For this review, take the finished solid that the model builds, in its own axes (mm). Face numbers are marked on the shaded views. A direction names the side the tool comes from. Give positions to 0.01 mm unless a question says otherwise; leave off trailing zeros. Order: outer loops, then holes, each group sorted by start corner. A loop starts at its lowest first (then second) coordinate and runs counter-clockwise, first axis right, second up.
Item 1: For probe 1 along Y at (x, z) = (0, -24.1); probe 2 along Y at (x, z) = (0, -6.5); probe 3 along Y at (x, z) = (0, -5), list the stretches that pass through material, from the lowest coordinate up.
Item 2: Consider section D-D (z = -20.25). Give the boundary of the cut face in (x, y).
Item 3: For P1, Ø3, axis at x = -0.5, z = -3.5, coming from the -Y side; P2, Ø3, axis at x = 3.5, z = -20, coming from the -Y side; P3, Ø1.5, axis at y = 4.5, z = -18.5, coming from the -X side, all flat-tipped, find the tip position at first contact; note any pin that passes through.
Item 4: Consider section A-A (z = -4.05). Give the boundary of the cut face in (x, y), plus the area to 3 significant figures.
Item 5: Machinability: for the marked faces 4 and 5, which of the approach directions +Z, -Z, +X, -X, +Y, -Y give a long, thin tool a straight path to every point of the face, cutting with its end or side? Answer none if there is none.
Item 6: Consider section C-C (z = -9). Give the boundary of the cut face in (x, y), plus the area to 3 significant figures.
Item 7: The part is to be moulded in two halves that separate along X. For the marked faces 1, 2 and 3, say which applies: released by +X, released by -X, zero draft, split by the parting line, or undercut.
Item 8: Consider section B-B (z = -24.75). Give the boundary of the cut face in (x, y).
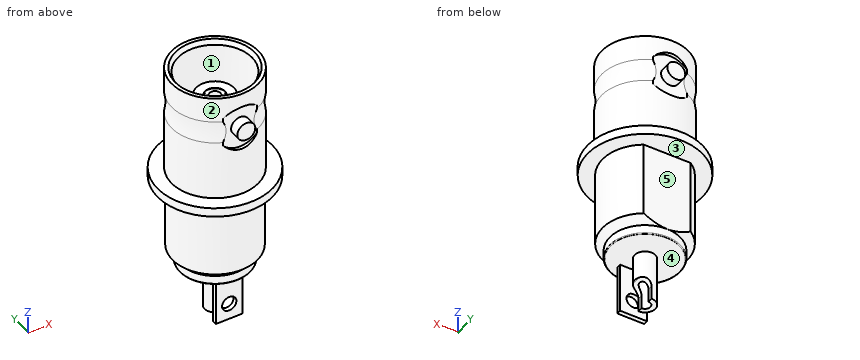
```python
from build123d import *

# Parameters (mm, degrees)
CUT_EXTRUDE_START        = 4.4
SKETCH_3_R               = 2.5
CUT_EXTRUDE_2_DEPTH      = 21.197865761
CUT_EXTRUDE_START_2      = -4.4
SKETCH_3_2_R             = 2.5
CUT_EXTRUDE_3_DEPTH      = 21.197865761
EXTRUDE_START            = 4.4
SKETCH_5_R               = 1
EXTRUDE_4_DEPTH          = 1.1
EXTRUDE_START_2          = -5.5
SKETCH_5_2_R             = 1
EXTRUDE_5_DEPTH          = 1.1
CUT_EXTRUDE_6_DEPTH      = 10
SKETCH_7_R               = 1.15
SKETCH_7_R_2             = 0.6
SKETCH_7_W               = 3
SKETCH_7_H               = 0.5
EXTRUDE_8_DEPTH          = 5.5
CUT_EXTRUDE_9_DEPTH      = 1.5
CUT_EXTRUDE_9_DEPTH_BACK = 1.5
SKETCH_9_R               = 0.8
CUT_EXTRUDE_10_DEPTH     = 1


with BuildPart() as part:
    # Эскиз1 → Повернуть1 (revolve)
    with BuildSketch(Plane(origin=(0, 0, 0), x_dir=(0, 0, -1), z_dir=(1, 0, 0)), mode=Mode.PRIVATE) as revolve_1_sk:
        with BuildLine():
            Line((10.3, 0), (10.3, 0.6))
            Line((10.3, 0.6), (3.3, 0.6))
            Line((3.3, 0.6), (3.3, 1))
            ThreePointArc((3.3, 1), (3.35, 1.05), (3.3, 1.1))
            Line((3.3, 1.1), (3.3, 2.1))
            Line((3.3, 2.1), (8.4, 2.1))
            Line((8.4, 2.1), (8.4, 4.1))
            Line((8.4, 4.1), (0.5, 4.1))
            Line((0.5, 4.1), (0, 4.4))
            Line((0, 4.4), (0, 4.8))
            Line((0, 4.8), (2.8, 4.8))
            ThreePointArc((2.8, 4.8), (4.05, 4.668347297), (5.3, 4.8))
            Line((5.3, 4.8), (11.9, 4.8))
            Line((11.9, 4.8), (11.9, 6.35))
            Line((11.9, 6.35), (12.9, 6.35))
            Line((12.9, 6.35), (12.9, 4.7))
            Line((12.9, 4.7), (21.1, 4.7))
            Line((21.1, 4.7), (21.9, 3.9))
            Line((21.9, 3.9), (22.8, 3.9))
            ThreePointArc((22.8, 3.9), (22.870710678, 3.870710678), (22.9, 3.8))
            Line((22.9, 3.8), (22.9, 0))
            Line((22.9, 0), (10.3, 0))
        make_face()
    revolve(revolve_1_sk.sketch.rotate(Axis((0, 0, 0), (0, 0, -1)), 90), axis=Axis((0, 0, 0), (0, 0, -1)))

    # Эскиз3 → Вытянуть2 (cut, through all)
    with BuildSketch(Plane(origin=(0, 0, 0), x_dir=(1, 0, 0), z_dir=(0, 1, 0)).offset(CUT_EXTRUDE_START)):
        with Locations((0, 4.05)):
            Circle(SKETCH_3_R)
    extrude(amount=CUT_EXTRUDE_2_DEPTH, mode=Mode.SUBTRACT)

    # Эскиз3<2> → Вытянуть3 (cut, through all)
    with BuildSketch(Plane(origin=(0, 0, 0), x_dir=(1, 0, 0), z_dir=(0, 1, 0)).offset(CUT_EXTRUDE_START_2)):
        with Locations((0, 4.05)):
            Circle(SKETCH_3_2_R)
    extrude(amount=-CUT_EXTRUDE_3_DEPTH, mode=Mode.SUBTRACT)

    # Эскиз5 → Вытянуть4 (add)
    with BuildSketch(Plane(origin=(0, 0, 0), x_dir=(1, 0, 0), z_dir=(0, 1, 0)).offset(EXTRUDE_START)):
        with Locations(Location((0, 4.05, 0), (0, 0, 270))):
            Circle(SKETCH_5_R)
    extrude(amount=EXTRUDE_4_DEPTH)

    # Эскиз5<2> → Вытянуть5 (add)
    with BuildSketch(Plane(origin=(0, 0, 0), x_dir=(1, 0, 0), z_dir=(0, 1, 0)).offset(EXTRUDE_START_2)):
        with Locations(Location((0, 4.05, 0), (0, 0, 270))):
            Circle(SKETCH_5_2_R)
    extrude(amount=EXTRUDE_5_DEPTH)

    # Эскиз2 → Вытянуть6 (cut)
    with BuildSketch(Plane(origin=(0, 0, -22.9), x_dir=(-1, 0, 0), z_dir=(0, 0, -1))):
        with BuildLine():
            Line((-2.62297541, 3.9), (2.62297541, 3.9))
            ThreePointArc((2.62297541, 3.9), (0, 4.7), (-2.62297541, 3.9))
        make_face()
    extrude(amount=-CUT_EXTRUDE_6_DEPTH, mode=Mode.SUBTRACT)

    # Эскиз7 → Вытянуть8 (add)
    # profile 1 of 2: a face of its own
    with BuildSketch(Plane(origin=(0, 0, -22.9), x_dir=(-1, 0, 0), z_dir=(0, 0, -1))):
        with Locations(Location((0, 0, 0), (0, 0, 180))):
            Circle(SKETCH_7_R)
        with Locations(Location((0, 0, 0), (0, 0, 180))):
            Circle(SKETCH_7_R_2, mode=Mode.SUBTRACT)
    # profile 2 of 2: a face of its own
    with BuildSketch(Plane(origin=(0, 0, -22.9), x_dir=(-1, 0, 0), z_dir=(0, 0, -1))):
        with Locations((0, -2.25)):
            Rectangle(SKETCH_7_W, SKETCH_7_H)
    extrude(amount=EXTRUDE_8_DEPTH)

    # Эскиз8 → Вытянуть9 (cut, two sides: drawn at the far end of the back side and taken through both)
    with BuildSketch(Plane(origin=(0, 0, 0), x_dir=(1, 0, 0), z_dir=(0, 1, 0)).offset(-CUT_EXTRUDE_9_DEPTH_BACK)):
        with BuildLine():
            Line((0, 30.676927372), (3.471261933, 30.676927372))
            Line((3.471261933, 30.676927372), (3.471261933, 25.9))
            Line((3.471261933, 25.9), (1, 25.9))
            ThreePointArc((1, 25.9), (0.292893219, 26.192893219), (0, 26.9))
            Line((0, 26.9), (0, 30.676927372))
        make_face()
    extrude(amount=CUT_EXTRUDE_9_DEPTH + CUT_EXTRUDE_9_DEPTH_BACK, mode=Mode.SUBTRACT)

    # Эскиз9 → Вытянуть10 (cut)
    with BuildSketch(Plane.XZ.offset(2.5)):
        with Locations((0, -26.6)):
            Circle(SKETCH_9_R)
    extrude(amount=-CUT_EXTRUDE_10_DEPTH, mode=Mode.SUBTRACT)


solid = part.part
```
Resolved:
1. probe 1: y = -2.5 to -2, -1.15 to -0.6, 0.6 to 1.15
1. probe 2: y = -4.4 to -4.1, -2.1 to -0.6, 0.6 to 2.1, 4.1 to 4.4
1. probe 3: y = -5.5 to -4.1, -2.1 to -0.6, 0.6 to 2.1, 4.1 to 5.5
2. outline: (-2.62, 3.9) arc R4.7 ccw (long way) to (2.62, 3.9) - close
3. P1: stops at y = -5.5
3. P2: stops at y = -4.25
3. P3: stops at x = -2.83
4. outline: circle Ø4.2 at (0, 0); (-1.56, -4.4) - (-1, -4.4) - (-1, -5.5) - (1, -5.5) - (1, -4.4) - (1.56, -4.4) arc R4.67 ccw to (1.56, 4.4) - (1, 4.4) - (1, 5.5) - (-1, 5.5) - (-1, 4.4) - (-1.56, 4.4) arc R4.67 ccw to start; hole circle Ø8.2 at (0, 0); hole circle Ø1.2 at (0, 0)
4. area: 31.7 mm2
5. face 4: -Z
5. face 5: -Z, +X, -X, +Y
6. outline: circle Ø9.6 at (0, 0); hole circle Ø1.2 at (0, 0)
6. area: 71.3 mm2
7. face 1: undercut
7. face 2: split by the parting line
7. face 3: zero draft
8. outline: (-1.5, -2.5) - (1.5, -2.5) - (1.5, -2) - (-1.5, -2) - close; circle Ø2.3 at (0, 0); hole circle Ø1.2 at (0, 0)
